CAD build for the part. Positions are in the model's coordinates, mm. A direction names the side the tool comes from. Give positions to 0.01 mm unless a question says otherwise; leave off trailing zeros. Write each loop counter-clockwise with the first axis right and the second up, starting at its lowest first coordinate (ties: lowest second). Pieces come first, ordered by that corner, then holes. Notation, with made-up numbers: (63.25, 32.5) - (115.25, 32.5) arc R29 ccw to (115.25, 63.5) - close; hole circle Ø6 at (29.25, 6). An arc over 180 degrees is marked (long way). Write item = value, one per line. Start each with the question number.
```python
from build123d import *

# Parameters (mm, degrees)
F1_DEPTH = 10
F0_W     = 30
F0_H     = 5
F2_DEPTH = 35
F4_DEPTH = 10.001
F6_DEPTH = 10.001


with BuildPart() as f1:
    # F0 (on Front) → F1 (new body)
    with BuildSketch(Plane.XZ):
        Polygon((-7.5, 20), (-32.5, 20), (-32.5, 15), (-22.5, 15), (-22.5, -10), (7.5, -10), (7.5, -15), (-22.5, -15), (-22.5, -20), (32.5, -20), (32.5, 0), align=None)
    extrude(amount=F1_DEPTH)

    # F0 (on Front) → F2 (join)
    with BuildSketch(Plane.XZ):
        Polygon((-22.5, 15), (-32.5, 15), (-32.5, -20), (-22.5, -20), (-22.5, -15), (-22.5, -10), align=None)
        with Locations((-7.5, -12.5)):
            Rectangle(F0_W, F0_H)
    extrude(amount=F2_DEPTH)

    # F3 (on face) → F4 (cut, through all)
    with BuildSketch(Plane.XY.offset(-10)):
        Polygon((7.5, -10), (-22.5, -35), (7.5, -35), align=None)
    extrude(amount=-F4_DEPTH, mode=Mode.SUBTRACT)

    # F5 (on face) → F6 (cut, through all)
    with BuildSketch(Plane.YZ.offset(-22.5)):
        Polygon((-35, 15), (-35, -10), (-10, 15), align=None)
    extrude(amount=-F6_DEPTH, mode=Mode.SUBTRACT)


solid = f1.part
```
1. Cut at A-A (y = -19.5). Give the cut face in (x, z), then the cut area to 3 significant figures.
2. Wall check: line 1 along Y through (x, z) = (-1, -8); line 2 along Z through (x, y) = (-18, -14.5); line 3 along X through (y, z) = (-26.5, -9.5). Give the ranges that are in metal, low to high.
3. Pin check, flat tips, straight feed: pin 1 Ø12.5 at (y, z) = (-19, 3) entering from +X; pin 2 Ø5 at (x, y) = (8.5, -7) entering from +Z; pin 3 Ø1 at (x, y) = (-21, -23.5) entering from +Z. Stop position of each tip, or through.
4. Tool access for faces 1 (the flat face through (-22.5, -22, -18)), 2 (the flat face through (-32.5, -13, -4)), 3 (the flat face through (-11, -20, -10)): list every direction of +Z, -Z, +X, -X, +Y, -Y with a clear straight run to the whole face (end or side of a thin tool).
5. Cut at C-C (z = 8). Give the cut face in (x, y), then the cut area to 3 significant figures.
6. Cut at D-D (y = -1.5). Give the cut face in (x, z).
7. Cut at B-B (x = -18). Give the cut face in (y, z).
Output:
q1.outline = (-32.5, -20) - (-22.5, -20) - (-22.5, -15) - (-3.9, -15) - (-3.9, -10) - (-22.5, -10) - (-22.5, 5.5) - (-32.5, 5.5) - close
q1.area = 348 mm2
q2.line_1 = -10 to 0
q2.line_2 = -15 to -10
q2.line_3 = -32.5 to -22.5
q3.pin_1 = -22.5
q3.pin_2 = 13.25
q3.pin_3 = -10
q4.face_1 = -Z, +X, -Y
q4.face_2 = +Z, -Z, -X, +Y, -Y
q4.face_3 = +Z, +X, -Y
q5.outline = (-32.5, -17) - (-22.5, -17) - (-22.5, -10) - (16.5, -10) - (16.5, 0) - (-32.5, 0) - close
q5.area = 560 mm2
q6.outline = (-32.5, -20) - (32.5, -20) - (32.5, 0) - (-7.5, 20) - (-32.5, 20) - close
q7.outline = (-31.25, -15) - (-10, -15) - (-10, -20) - (0, -20) - (0, 20) - (-10, 20) - (-10, -10) - (-31.25, -10) - close
